from build123d import *

# Parameters (mm, degrees)
SKETCH1_W           = 11.9
SKETCH1_H           = 5.95
BOSS_EXTRUDE1_DEPTH = 290
CUT_EXTRUDE1_DEPTH  = 291


with BuildPart() as part:
    # Sketch1 → Boss-Extrude1 (new body)
    with BuildSketch(Plane.XY):
        with BuildLine():
            Line((-4.350229073, 14.992640687), (-13.192640687, 14.992640687))
            ThreePointArc((-13.192640687, 14.992640687), (-14.465432893, 14.465432893), (-14.992640687, 13.192640687))
            Line((-14.992640687, 13.192640687), (-14.992640687, 4.350229073))
            Line((-14.992640687, 4.350229073), (-13.792640687, 4.350229073))
            ThreePointArc((-13.792640687, 4.350229073), (-13.085533906, 4.643122292), (-12.792640687, 5.350229073))
            Line((-12.792640687, 5.350229073), (-12.792640687, 8.460229073))
            Line((-12.792640687, 8.460229073), (-8.460229073, 8.460229073))
            Line((-8.460229073, 8.460229073), (-8.460229073, 12.792640687))
            Line((-8.460229073, 12.792640687), (-5.350229073, 12.792640687))
            ThreePointArc((-5.350229073, 12.792640687), (-4.643122292, 13.085533906), (-4.350229073, 13.792640687))
            Line((-4.350229073, 13.792640687), (-4.350229073, 14.992640687))
        make_face()
        with BuildLine():
            Line((-10.660229073, 13.792640687), (-12.792640687, 13.792640687))
            ThreePointArc((-12.792640687, 13.792640687), (-13.499747468, 13.499747468), (-13.792640687, 12.792640687))
            Line((-13.792640687, 12.792640687), (-13.792640687, 10.660229073))
            ThreePointArc((-13.792640687, 10.660229073), (-13.499747468, 9.953122292), (-12.792640687, 9.660229073))
            Line((-12.792640687, 9.660229073), (-10.660229073, 9.660229073))
            ThreePointArc((-10.660229073, 9.660229073), (-9.953122292, 9.953122292), (-9.660229073, 10.660229073))
            Line((-9.660229073, 10.660229073), (-9.660229073, 12.792640687))
            ThreePointArc((-9.660229073, 12.792640687), (-9.953122292, 13.499747468), (-10.660229073, 13.792640687))
        make_face(mode=Mode.SUBTRACT)
        Polygon((-5.95, 4.217588386), (-5.95, 5.95), (-4.217588386, 5.95), (-8.460229073, 10.192640687), (-8.460229073, 8.460229073), (-10.192640687, 8.460229073), align=None)
        with Locations((0, 2.975)):
            Rectangle(SKETCH1_W, SKETCH1_H)
        Polygon((8.460229073, 10.192640687), (4.217588386, 5.95), (5.95, 5.95), (5.95, 4.217588386), (10.192640687, 8.460229073), (8.460229073, 8.460229073), align=None)
        with BuildLine():
            Line((12.792640687, 8.460229073), (12.792640687, 5.350229073))
            ThreePointArc((12.792640687, 5.350229073), (13.085533906, 4.643122292), (13.792640687, 4.350229073))
            Line((13.792640687, 4.350229073), (14.992640687, 4.350229073))
            Line((14.992640687, 4.350229073), (14.992640687, 13.192640687))
            ThreePointArc((14.992640687, 13.192640687), (14.465432893, 14.465432893), (13.192640687, 14.992640687))
            Line((13.192640687, 14.992640687), (4.350229073, 14.992640687))
            Line((4.350229073, 14.992640687), (4.350229073, 13.792640687))
            ThreePointArc((4.350229073, 13.792640687), (4.643122292, 13.085533906), (5.350229073, 12.792640687))
            Line((5.350229073, 12.792640687), (8.460229073, 12.792640687))
            Line((8.460229073, 12.792640687), (8.460229073, 8.460229073))
            Line((8.460229073, 8.460229073), (12.792640687, 8.460229073))
        make_face()
        with BuildLine():
            ThreePointArc((9.660229073, 10.660229073), (9.953122292, 9.953122292), (10.660229073, 9.660229073))
            Line((10.660229073, 9.660229073), (12.792640687, 9.660229073))
            ThreePointArc((12.792640687, 9.660229073), (13.499747468, 9.953122292), (13.792640687, 10.660229073))
            Line((13.792640687, 10.660229073), (13.792640687, 12.792640687))
            ThreePointArc((13.792640687, 12.792640687), (13.499747468, 13.499747468), (12.792640687, 13.792640687))
            Line((12.792640687, 13.792640687), (10.660229073, 13.792640687))
            ThreePointArc((10.660229073, 13.792640687), (9.953122292, 13.499747468), (9.660229073, 12.792640687))
            Line((9.660229073, 12.792640687), (9.660229073, 10.660229073))
        make_face(mode=Mode.SUBTRACT)
    extrude(amount=-BOSS_EXTRUDE1_DEPTH)

    # Mirror1: part across plane


with BuildPart() as part_1:
    add(part.part)
    add(part.part.mirror(Plane(origin=(0, 0, -290), x_dir=(0, 0, 1), z_dir=(0, -1, 0))))

    # Sketch2 → Cut-Extrude1 (cut, through all)
    with BuildSketch(Plane.XY):
        with BuildLine():
            Line((-4.631549417, 3.075914498), (-3.16821753, 1.612582612))
            ThreePointArc((-3.16821753, 1.612582612), (-2.513764607, 2.513764607), (-1.612582612, 3.16821753))
            Line((-1.612582612, 3.16821753), (-3.075914498, 4.631549417))
            Line((-3.075914498, 4.631549417), (-4.631549417, 3.075914498))
        make_face()
        with BuildLine():
            Line((-3.16821753, 1.612582612), (-1.555634919, 0))
            Line((-1.555634919, 0), (0, 1.555634919))
            Line((0, 1.555634919), (-1.612582612, 3.16821753))
            ThreePointArc((-1.612582612, 3.16821753), (-2.513764607, 2.513764607), (-3.16821753, 1.612582612))
        make_face()
        with BuildLine():
            ThreePointArc((-3.16821753, 1.612582612), (-3.555, 0), (-3.16821753, -1.612582612))
            Line((-3.16821753, -1.612582612), (-1.555634919, 0))
            Line((-1.555634919, 0), (-3.16821753, 1.612582612))
        make_face()
        with BuildLine():
            Line((-4.631549417, -3.075914498), (-3.075914498, -4.631549417))
            Line((-3.075914498, -4.631549417), (-1.612582612, -3.16821753))
            ThreePointArc((-1.612582612, -3.16821753), (-2.513764607, -2.513764607), (-3.16821753, -1.612582612))
            Line((-3.16821753, -1.612582612), (-4.631549417, -3.075914498))
        make_face()
        with BuildLine():
            ThreePointArc((-3.16821753, -1.612582612), (-2.513764607, -2.513764607), (-1.612582612, -3.16821753))
            Line((-1.612582612, -3.16821753), (0, -1.555634919))
            Line((0, -1.555634919), (-1.555634919, 0))
            Line((-1.555634919, 0), (-3.16821753, -1.612582612))
        make_face()
        with BuildLine():
            Line((0, -1.555634919), (-1.612582612, -3.16821753))
            ThreePointArc((-1.612582612, -3.16821753), (0, -3.555), (1.612582612, -3.16821753))
            Line((1.612582612, -3.16821753), (0, -1.555634919))
        make_face()
        with BuildLine():
            Line((1.555634919, 0), (0, -1.555634919))
            Line((0, -1.555634919), (1.612582612, -3.16821753))
            ThreePointArc((1.612582612, -3.16821753), (2.513764607, -2.513764607), (3.16821753, -1.612582612))
            Line((3.16821753, -1.612582612), (1.555634919, 0))
        make_face()
        with BuildLine():
            Line((3.16821753, 1.612582612), (1.555634919, 0))
            Line((1.555634919, 0), (3.16821753, -1.612582612))
            ThreePointArc((3.16821753, -1.612582612), (3.456952294, -0.829159719), (3.555, 0))
            ThreePointArc((3.555, 0), (3.456952294, 0.829159719), (3.16821753, 1.612582612))
        make_face()
        Polygon((-1.555634919, 0), (0, -1.555634919), (1.555634919, 0), (0, 1.555634919), align=None)
        with BuildLine():
            Line((0, 1.555634919), (1.555634919, 0))
            Line((1.555634919, 0), (3.16821753, 1.612582612))
            ThreePointArc((3.16821753, 1.612582612), (2.513764607, 2.513764607), (1.612582612, 3.16821753))
            Line((1.612582612, 3.16821753), (0, 1.555634919))
        make_face()
        with BuildLine():
            Line((-1.612582612, 3.16821753), (0, 1.555634919))
            Line((0, 1.555634919), (1.612582612, 3.16821753))
            ThreePointArc((1.612582612, 3.16821753), (0, 3.555), (-1.612582612, 3.16821753))
        make_face()
        with BuildLine():
            ThreePointArc((1.612582612, 3.16821753), (2.513764607, 2.513764607), (3.16821753, 1.612582612))
            Line((3.16821753, 1.612582612), (4.631549417, 3.075914498))
            Line((4.631549417, 3.075914498), (3.075914498, 4.631549417))
            Line((3.075914498, 4.631549417), (1.612582612, 3.16821753))
        make_face()
        with BuildLine():
            ThreePointArc((3.16821753, -1.612582612), (2.513764607, -2.513764607), (1.612582612, -3.16821753))
            Line((1.612582612, -3.16821753), (3.075914498, -4.631549417))
            Line((3.075914498, -4.631549417), (4.631549417, -3.075914498))
            Line((4.631549417, -3.075914498), (3.16821753, -1.612582612))
        make_face()
    extrude(amount=-CUT_EXTRUDE1_DEPTH, mode=Mode.SUBTRACT)


solid = part_1.part
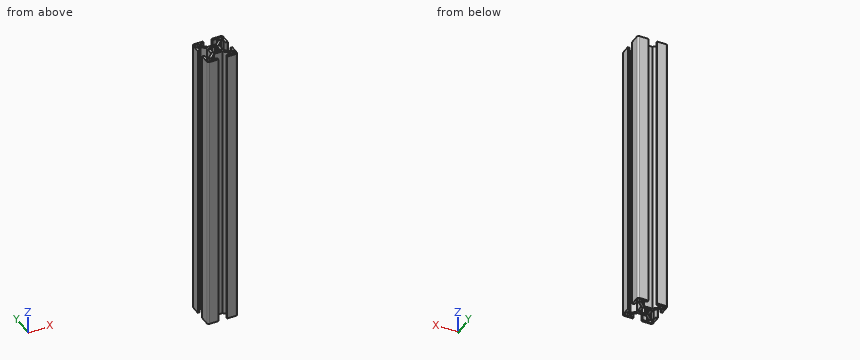
Source: CAD feature listing. Evaluate the final solid. Frame: model axes, mm. Round coordinates to 2 decimals unless told otherwise and drop trailing zeros. Return JSON: item names as keys, results as strings. Group by question number.
1. Material intervals for line 1 along Y through (x, z) = (10.5, -140.5); line 2 along X through (y, z) = (-12.5, -238.5); line 3 along Y through (x, z) = (-4.5, -228), sorted ascending. Write a range as from..to.
2. Section query A-A on z = -217. State how many separate pieces and enclosed holes the cut face has, and give its area (3 significant figures).
3. Pin query (flat end, axial travel): pin 1 (1 mm diameter, centred on y = -3.5, z = -199.5, fed in from -X); pin 2 (2.5 mm diameter, centred on x = 0.5, z = -217, fed in from -Y); pin 3 (2 mm diameter, centred on x = -7.5, y = -2.5, fed in from -Z). Return the tip coordinate at first contact, or that it passes through.
Checks:
{
 "1": {"line 1": "y = -14.99..-13.78, -9.67..-8.46, 8.46..9.67, 13.78..14.99", "line 2": "x = -14.99..-13.79, -9.66..-8.46, 8.46..9.66, 13.79..14.99", "line 3": "y = -14.99..-13.27, -6.23..-3.21, -2.94..2.94, 3.21..6.23, 13.27..14.99"},
 "2": {"separate pieces": "1", "enclosed holes": "5", "area": "305 mm²"},
 "3": {"pin 1": "stops at x = -5.95", "pin 2": "stops at y = -5.95", "pin 3": "passes through"}
}
